Here's the drawing with two shaded views (mm, measured from the low corner). I have some questions. A direction names the side the tool comes from. Give positions to 0.01 mm unless a question says otherwise; leave off trailing zeros. Loops run counter-clockwise (first coordinate to the right, second up) from the corner with the lowest first, then second, coordinate; pieces in that order, holes last. Notation, with made-up numbers: M 78.25,81 L 107.25,81 A18 ccw 107.25,89 Z; hole C 42,44 d11. An arc over 180 degrees is marked long. Use CSV: the item, a comma, the result in double quotes.
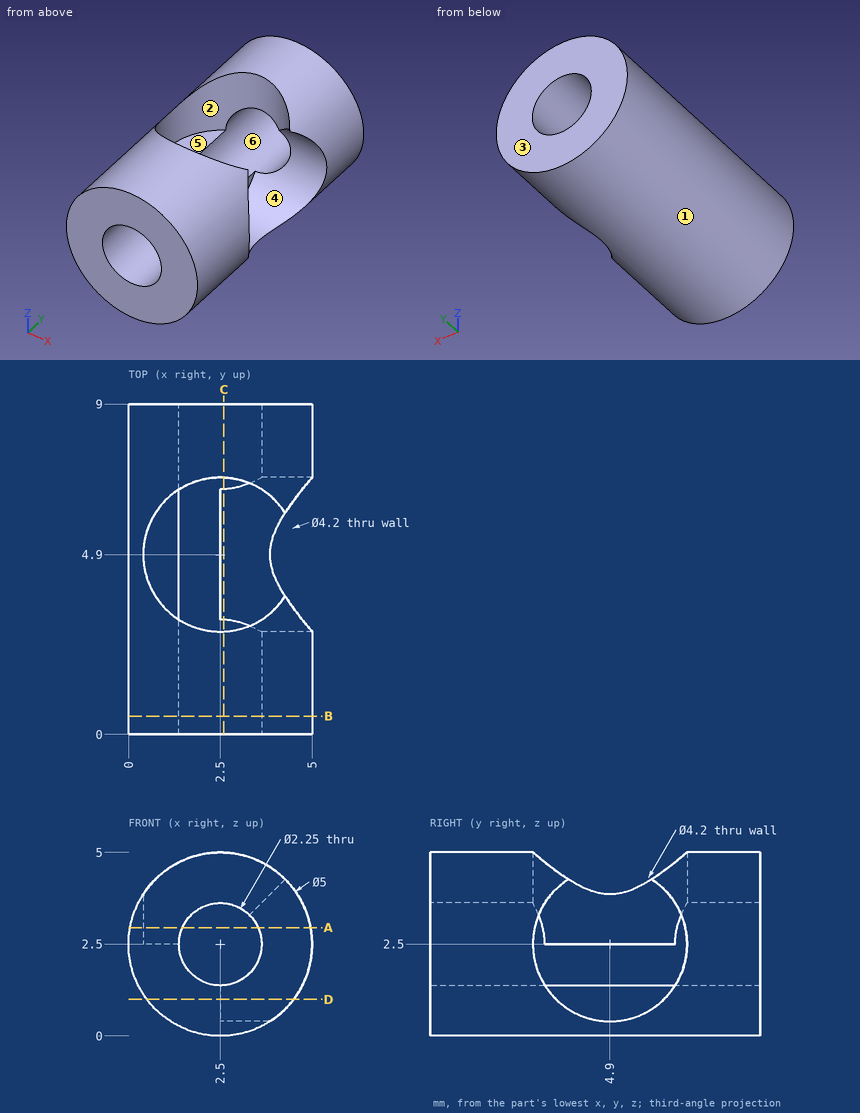
1. I want a section at D-D, the plane z = 1. List the corners of the cut face in (x, y) for me, then the cut area to 3 significant figures.
Outcome:
outline,"M 0.5,0 L 4.5,0 L 4.5,3.43 L 2.5,3.43 L 2.5,6.37 L 4.5,6.37 L 4.5,9 L 0.5,9 Z"
area,"30.1 mm2"
2. Please list where these lines run through material, in increasing order: line 1 (Z direction, x = 2.5, y = 2) (3 decimals); line 2 (Y direction, x = 2.45, z = 4.5); line 3 (Y direction, x = 4.65, z = 1.3).
Outcome:
line 1,"0 to 1.375, 3.625 to 5"
line 2,"0 to 2.8, 7 to 9"
line 3,"0 to 3.18, 6.62 to 9"
3. I want a section at C-C, the plane x = 2.6. List the corners of the cut face in (y, z) for me, then the cut area to 3 significant figures.
Outcome:
outline,"M 0,0 L 9,0 L 9,1.38 L 6.68,1.38 A2.1 cw 3.12,1.38 L 0,1.38 Z; M 0,3.62 L 2.8,3.62 L 2.8,5 L 0,5 Z; M 7,3.62 L 9,3.62 L 9,5 L 7,5 Z"
area,"16.6 mm2"
4. If we mould it in two halves opening along X, with no side actions, what happens to the marked faces 1, 2 and 3? For each: +X half, -X half, draft (parallel to the pull), parting line (faces both ways), or undercut.
Outcome:
face 1,"parting line"
face 2,"undercut"
face 3,"draft"
5. I want a section at B-B, the plane y = 0.5. List the corners of the cut face in (x, z) for me (3 decimals), then the cut area to 3 significant figures.
Outcome:
outline,"C 2.5,2.5 d5; hole C 2.5,2.5 d2.25"
area,"15.7 mm2"
6. I want a section at A-A, the plane z = 2.95. List the corners of the cut face in (x, y) for me, then the cut area to 3 significant figures.
Outcome:
outline,"M 0.04,0 L 1.47,0 L 1.47,3.07 A2.1 cw 1.47,6.73 L 1.47,9 L 0.04,9 Z; M 3.53,0 L 4.96,0 L 4.96,2.85 L 3.53,2.85 Z; M 3.53,6.95 L 4.96,6.95 L 4.96,9 L 3.53,9 Z"
area,"17.1 mm2"
7. I'm going to push flat-ended pins straight in: pin 1 Ø2 at (y, z) = (3.5, 1) entering from +X; pin 2 Ø1.1 at (y, z) = (5, 1) entering from +X; pin 3 Ø2 at (y, z) = (2, 0.5) entering from +X; pin 4 Ø3 at (x, z) = (2.5, 2.5) entering from -Y. Where does each tip first touch, or does it pass through?
Outcome:
pin 1,"x = 4.9"
pin 2,"x = 2.5"
pin 3,"x = 4.79"
pin 4,"y = 0"
8. Which directions (+Z, -Z, +X, -X, +Y, -Y) give clear straight access to the entire face, cutting with the end or side of a thin tool? Please do the marked faces 4, 5 and 6.
Outcome:
face 4,"+X"
face 5,"+Z, +X"
face 6,"+Y, -Y"
